from build123d import *

# Parameters (mm, degrees)
SKETCH3_W               = 20
SKETCH3_H               = 10
BOSS_EXTRUDE1_DEPTH     = 40
CUT_EXTRUDE1_DEPTH      = 83.462112512
CUT_EXTRUDE1_DEPTH_BACK = 83.462112512
SKETCH4_R               = 4
SKETCH7_W               = 90
SKETCH7_H               = 40
BOSS_EXTRUDE3_DEPTH     = 20
SKETCH8_R               = 1.5
CUT_EXTRUDE3_DEPTH      = 20


with BuildPart() as part:
    # Sketch3 → Boss-Extrude1 (new body)
    with BuildSketch(Plane(origin=(0, 0, 0), x_dir=(1, 0, 0), z_dir=(0, 1, 0))):
        with Locations((-35, 35)):
            Rectangle(SKETCH3_W, SKETCH3_H)
        Polygon((-25, 30), (-25, 0), (-15, 0), (-15, 30), (0, 30), (0, 40), (-25, 40), align=None)
        Polygon((0, 40), (0, 30), (15, 30), (15, 0), (25, 0), (25, 30), (25, 40), align=None)
        with Locations((35, 35)):
            Rectangle(SKETCH3_W, SKETCH3_H)
    extrude(amount=BOSS_EXTRUDE1_DEPTH)

    # Sketch4 → Cut-Extrude1 (cut, two sides: drawn at the far end of the back side and taken through both)
    with BuildSketch(Plane(origin=(-15, 0, 0), x_dir=(0, 0, -1), z_dir=(1, 0, 0)).offset(-CUT_EXTRUDE1_DEPTH_BACK)):
        with Locations((15, 20)):
            Circle(SKETCH4_R)
    extrude(amount=CUT_EXTRUDE1_DEPTH + CUT_EXTRUDE1_DEPTH_BACK, mode=Mode.SUBTRACT)

    # Sketch7 → Boss-Extrude3 (add)
    with BuildSketch(Plane.XZ):
        with Locations((0, -20)):
            Rectangle(SKETCH7_W, SKETCH7_H)
    extrude(amount=BOSS_EXTRUDE3_DEPTH)

    # Sketch8 → Cut-Extrude3 (cut)
    with BuildSketch(Plane.XZ.offset(20)):
        with Locations(Location((-24.25, -5, 0), (0, 0, 270))):
            Circle(SKETCH8_R)
        with Locations(Location((24.25, -5, 0), (0, 0, 270))):
            Circle(SKETCH8_R)
    extrude(amount=-CUT_EXTRUDE3_DEPTH, mode=Mode.SUBTRACT)


solid = part.part
Input: part model. Units: mm. Frame: model coordinates. A direction names the side the tool comes from. Give positions to 0.01 mm unless a question says otherwise; leave off trailing zeros. Order: outer loops, then holes, each group sorted by start corner. A loop starts at its lowest first (then second) coordinate and runs counter-clockwise, first axis right, second up. Notation, with made-up numbers: (68.5, -14) - (85.5, -14) arc R19 ccw to (85.5, -9) - close; hole circle Ø10 at (-21.75, 72). An arc over 180 degrees is marked (long way). Answer as a JSON object with one key per item and string values. Group by question number.
Q1. Line query: probe 1 along X at (y, z) = (4, -21); probe 2 along X at (y, z) = (-12, -5); probe 3 along Z at (x, y) = (-21, 20). Output: solid intervals per line, ascending.
Q2. Cut plane B-B, the plane z = -26.5. Output: boundary loops of the cut face in (x, y).
Q3. Set-up query: faces 1 (the face through (0, 0, -15)), 2 (the face through (-25, 15, -15)), 3 (the face through (35, 20, -30)), 4 (the face through (24, 0, -5)). Return all of +Z, -Z, +X, -X, +Y, -Y with unobstructed straight access to the full face (end or side cutting, diameter ignored); none if empty.
Q4. Mould query, pull axis Z, two halves, no side actions, for faces 5 (the face through (35, 0, -15)), 6 (the face through (25.737, -10.14, -4.805)), 7 (the face through (-1, 10, -40)). Classes: pulls with the +Z half, pulls with the -Z half, needs draft (parallel to the pull), parting line crosses it, or undercut.
Q5. Cut plane C-C, the plane x = -21. Output: boundary loops of the cut face in (y, z).
Q6. First-contact query: pin 1 Ø12 at (y, z) = (10, -22.5) entering from +X; pin 2 Ø4 at (x, z) = (1, -27.5) entering from +Y; pin 3 Ø1.8 at (x, z) = (24, -5) entering from -Y; pin 4 Ø3.5 at (x, z) = (-24.25, -5) entering from -Y. Flat tips, straight axial feed; report the tip coordinate or a pass-through.
Q7. Cut plane A-A, the plane y = 20. Output: boundary loops of the cut face in (x, z), then the cut area to 3 significant figures.
Q8. Cut plane D-D, the plane z = -15. Output: boundary loops of the cut face in (x, y).
Results:
{
 "1": {"probe 1": "-25 to -15, 15 to 25", "probe 2": "-45 to -25.75, -22.75 to 22.75, 25.75 to 45", "probe 3": "-40 to -19, -11 to 0"},
 "2": {"outline": "(-45, -20) - (45, -20) - (45, 0) - (25, 0) - (25, 40) - (15, 40) - (15, 0) - (-15, 0) - (-15, 40) - (-25, 40) - (-25, 0) - (-45, 0) - close"},
 "3": {"face 1": "+Z, +Y", "face 2": "+Z, -X, +Y", "face 3": "+Z, +X, +Y", "face 4": "-Y"},
 "4": {"face 5": "needs draft", "face 6": "undercut", "face 7": "pulls with the -Z half"},
 "5": {"outline": "(-20, -40) - (40, -40) - (40, 0) - (-20, 0) - close; hole circle Ø8 at (20, -15)"},
 "6": {"pin 1": "x = 25", "pin 2": "y = 0", "pin 3": "y = 0", "pin 4": "y = -20"},
 "7": {"outline": "(-45, -40) - (45, -40) - (45, -30) - (25, -30) - (25, -19) - (15, -19) - (15, -30) - (-15, -30) - (-15, -19) - (-25, -19) - (-25, -30) - (-45, -30) - close; (-25, -11) - (-15, -11) - (-15, 0) - (-25, 0) - close; (15, -11) - (25, -11) - (25, 0) - (15, 0) - close", "area": "1,340 mm^2"},
 "8": {"outline": "(-45, -20) - (45, -20) - (45, 0) - (25, 0) - (25, 16) - (15, 16) - (15, 0) - (-15, 0) - (-15, 16) - (-25, 16) - (-25, 0) - (-45, 0) - close; (-25, 24) - (-15, 24) - (-15, 40) - (-25, 40) - close; (15, 24) - (25, 24) - (25, 40) - (15, 40) - close"}
}
